For this review, take the finished solid that the model builds, in its own axes (mm). Coordinates: 2 decimals unless noted, no trailing zeros. Write each loop counter-clockwise with the first axis right and the second up, starting at its lowest first coordinate (ties: lowest second). Pieces come first, ordered by that corner, then holes. Notation, with made-up numbers: M 46,79 L 90,79 A18 cw 90,105 Z; hole C -5.5,76 d4. An arc over 180 degrees is marked long. Return JSON: item names as keys, results as strings.
```python
from build123d import *

# Parameters (mm, degrees)
BASE_FLANGE1_DEPTH = 6.35
SKETCH7_W          = 25.4
SKETCH7_H          = 5.55625
TAB1_DEPTH         = 6.35
SKETCH10_R         = 5.159375
CUT_EXTRUDE1_DEPTH = 397.478917898
CUT_EXTRUDE2_DEPTH = 397.478917898
SKETCH12_R         = 12.7
CUT_EXTRUDE4_DEPTH = 397.478917898
FILLET1_R          = 2.54
FILLET2_R          = 0.396875


# Sheet-metal steps are written as plain solids
with BuildPart() as part:
    # Sketch2 → Base-Flange1 (new body)
    with BuildSketch(Plane.XY):
        with BuildLine():
            Line((0, 9.226103289), (0, 96.818079958))
            ThreePointArc((0, 96.818079958), (5.235649853, 107.092975426), (16.62574439, 108.896098462))
            Line((16.62574439, 108.896098462), (59.799322894, 94.863297175))
            ThreePointArc((59.799322894, 94.863297175), (62.104900611, 93.851471549), (64.16555713, 92.40469084))
            Line((64.16555713, 92.40469084), (99.070578742, 62.316397702))
            ThreePointArc((99.070578742, 62.316397702), (101.131235261, 60.869616993), (103.436812978, 59.857791367))
            Line((103.436812978, 59.857791367), (251.828096727, 11.625852535))
            ThreePointArc((251.828096727, 11.625852535), (253.766485462, 11.160330172), (255.753841117, 11.003871039))
            Line((255.753841117, 11.003871039), (368.3, 11.003871039))
            ThreePointArc((368.3, 11.003871039), (377.280256121, 7.28412716), (381, -1.696128961))
            Line((381, -1.696128961), (381, -21.925343231))
            ThreePointArc((381, -21.925343231), (380.234096284, -26.268999051), (378.028764428, -30.088745874))
            Line((378.028764428, -30.088745874), (341.720264081, -73.359531604))
            ThreePointArc((341.720264081, -73.359531604), (337.358751578, -76.706237856), (331.991499654, -77.896128961))
            Line((331.991499654, -77.896128961), (239.656685085, -77.896128961))
            Line((239.656685085, -77.896128961), (8.77425561, -2.851915215))
            ThreePointArc((8.77425561, -2.851915215), (2.425104532, 1.761753142), (0, 9.226103289))
        make_face()
    extrude(amount=-BASE_FLANGE1_DEPTH)

    # Sketch7 → Tab1 (add)
    with BuildSketch(Plane.XY):
        with Locations((265.056685085, -80.674253961)):
            Rectangle(SKETCH7_W, SKETCH7_H)
    extrude(amount=-TAB1_DEPTH)

    # Sketch10 → Cut-Extrude1 (cut, through all)
    with BuildSketch(Plane.XY):
        with Locations((361.95, -8.046128961)):
            Circle(SKETCH10_R)
        with Locations((329.296389428, -46.961186671)):
            Circle(SKETCH10_R)
        with Locations((19.05, 91.122091624)):
            Circle(SKETCH10_R)
        with Locations((19.05, 14.922091624)):
            Circle(SKETCH10_R)
        with Locations((45.111934921, 86.526669328)):
            Circle(SKETCH10_R)
        with Locations((153.335293858, 14.922091624)):
            Circle(SKETCH10_R)
        with Locations((105.023219841, 30.625069183)):
            Circle(SKETCH10_R)
    extrude(amount=-CUT_EXTRUDE1_DEPTH, mode=Mode.SUBTRACT)

    # Sketch11 → Cut-Extrude2 (cut, through all)
    with BuildSketch(Plane.XY):
        with BuildLine():
            Line((270.98625, -20.349253961), (287.02, -20.349253961))
            ThreePointArc((287.02, -20.349253961), (290.612102448, -21.837151512), (292.1, -25.429253961))
            Line((292.1, -25.429253961), (292.1, -41.463003961))
            ThreePointArc((292.1, -41.463003961), (290.612102448, -45.055106409), (287.02, -46.543003961))
            Line((287.02, -46.543003961), (270.98625, -46.543003961))
            ThreePointArc((270.98625, -46.543003961), (267.394147552, -45.055106409), (265.90625, -41.463003961))
            Line((265.90625, -41.463003961), (265.90625, -25.429253961))
            ThreePointArc((265.90625, -25.429253961), (267.394147552, -21.837151512), (270.98625, -20.349253961))
        make_face()
    extrude(amount=-CUT_EXTRUDE2_DEPTH, mode=Mode.SUBTRACT)

    # Sketch12 → Cut-Extrude4 (cut, through all)
    with BuildSketch(Plane.XY):
        with Locations((237.551232799, -89.527827626)):
            Circle(SKETCH12_R)
    extrude(amount=-CUT_EXTRUDE4_DEPTH, mode=Mode.SUBTRACT)

    # Fillet1
    fillet1_edges = [part.edges().sort_by_distance(p)[0] for p in [
        (236.503199055, -76.871144598, -3.175),
        (242.649623344, -77.896128961, -3.175),
    ]]
    fillet(fillet1_edges, radius=FILLET1_R)

    # Fillet2
    fillet2_edges = [part.edges().sort_by_distance(p)[0] for p in [
        (252.356685085, -77.896128961, -3.175),
        (277.756685085, -77.896128961, -3.175),
        (277.756685085, -83.452378961, -3.175),
        (252.356685085, -83.452378961, -3.175),
    ]]
    fillet(fillet2_edges, radius=FILLET2_R)


solid = part.part
```
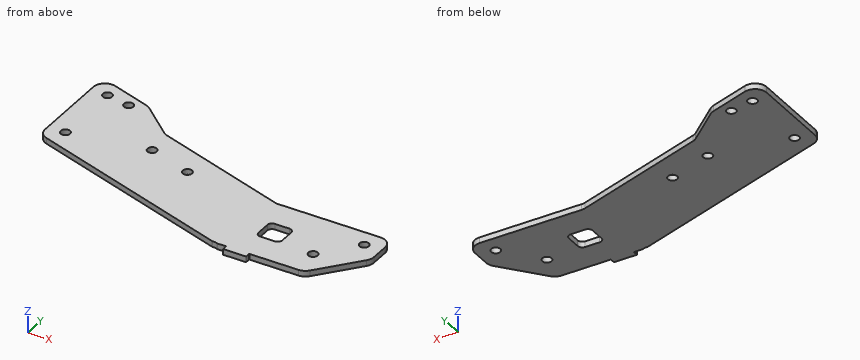
1. Clearance check with flat-ended pins moving along their axes: pin 1 Ø3 at (x, z) = (228.5, -1) entering from +Y; pin 2 Ø1.9 at (x, z) = (298.5, -3) entering from -Y; pin 3 Ø2.5 at (y, z) = (-79.5, -2.5) entering from -X. State where each tip first meets the part, or that it passes through.
Checks:
{"pin 1": "y = 19.7", "pin 2": "y = -77.9", "pin 3": "x = 252.35"}
2. We need section D-D (x = 203). State the section outline as (y, z) points, plus the area to 3 significant figures.
Checks:
{"outline": "M -65.98,-6.35 L 27.5,-6.35 L 27.5,0 L -65.98,0 Z", "area": "594 mm2"}
3. We need section C-C (z = -1.25). Give the number of separate pieces and of enclosed holes in the cut face, plus the area to 3 significant figures.
Checks:
{"separate pieces": "1", "enclosed holes": "8", "area": "34,400 mm2"}
4. We need section A-A (y = -37). State the section outline as (x, z) points.
Checks:
{"outline": "M 113.83,-6.35 L 265.91,-6.35 L 265.91,0 L 113.83,0 Z; M 292.1,-6.35 L 372.23,-6.35 L 372.23,0 L 292.1,0 Z"}
5. Wall thickness on L1, parallel to Y at x = 334.5, z = -2; L2, parallel to Y at x = 298.5, z = -5.5; L3, parallel to Y at x = 109, z = -1: over which ranges is each line inside the solid? List them lowest first. Write a range as from..to.
Checks:
{"L1": "-77.65..11", "L2": "-77.9..11", "L3": "-35.43..27.34, 33.91..58.05"}
6. We need section B-B (x = 361.95). State the section outline as (y, z) points.
Checks:
{"outline": "M -49.25,-6.35 L -13.21,-6.35 L -13.21,0 L -49.25,0 Z; M -2.89,-6.35 L 11,-6.35 L 11,0 L -2.89,0 Z"}
